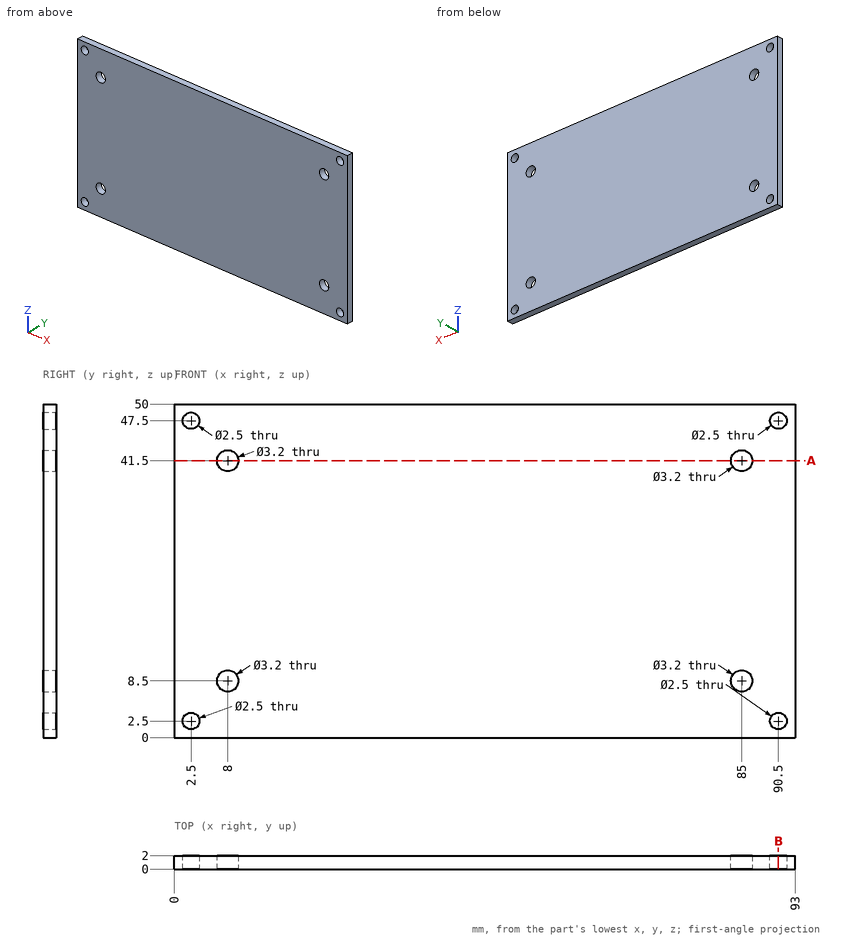
Geometry check sheet. Reference: drawing and pictorial views, mm from the part's lowest x, y, z. Coordinates: 2 decimals unless noted, no trailing zeros. Order: outer loops, then holes, each group sorted by start corner. A loop starts at its lowest first (then second) coordinate and runs counter-clockwise, first axis right, second up.
Item 1: Section check B-B (x = 90.5). Enter the section's corners in (y, z).
Item 2: Scan lines: line 1 along X through (y, z) = (0.75, 41.5); line 2 along Z through (x, y) = (8, 1.15); line 3 along Z through (x, y) = (2.5, 1.55). Record each from-to range of solid material in increasing order.
Item 3: Depth check by flat-ended pin: pin 1 (2.5 mm diameter, centred on x = 8, z = 41.5, fed in from +Y). Enter the tip coordinate at first touch or a pass-through.
Item 4: Section check A-A (z = 41.5). Enter the section's corners in (x, y).
Check sheet entries:
1. outline: (0, 0) - (2, 0) - (2, 1.25) - (0, 1.25) - close; (0, 3.75) - (2, 3.75) - (2, 46.25) - (0, 46.25) - close; (0, 48.75) - (2, 48.75) - (2, 50) - (0, 50) - close
2. line 1: x = 0 to 6.4, 9.6 to 83.4, 86.6 to 93
2. line 2: z = 0 to 6.9, 10.1 to 39.9, 43.1 to 50
2. line 3: z = 0 to 1.25, 3.75 to 46.25, 48.75 to 50
3. pin 1: passes through
4. outline: (0, 0) - (6.4, 0) - (6.4, 2) - (0, 2) - close; (9.6, 0) - (83.4, 0) - (83.4, 2) - (9.6, 2) - close; (86.6, 0) - (93, 0) - (93, 2) - (86.6, 2) - close
